from build123d import *

# Parameters (mm, degrees)
F1_DEPTH = 2.54
F2_R     = 1.651
F3_DEPTH = 25.4


with BuildPart() as f1:
    # F0 (on Front) → F1 (new body)
    with BuildSketch(Plane.XZ):
        with BuildLine():
            Line((-19.05, 0), (0, 0))
            Line((0, 0), (76.2, 0))
            ThreePointArc((76.2, 0), (100.04356, 25.4), (76.2, 50.8))
            Line((76.2, 50.8), (0, 50.8))
            Line((0, 50.8), (-19.05, 50.8))
            ThreePointArc((-19.05, 50.8), (-39.70724, 25.4), (-19.05, 0))
        make_face()
    extrude(amount=F1_DEPTH)

    # F2 (on face) → F3 (cut)
    with BuildSketch(Plane.XZ.offset(2.54)):
        with Locations((59.7933, 39.132159)):
            Circle(F2_R)
        with Locations((85.7267, 39.132159)):
            Circle(F2_R)
        with Locations((34.717675, 39.132159)):
            Circle(F2_R)
        with Locations((7.566978, 39.132159)):
            Circle(F2_R)
        with Locations((-13.534474, 39.132159)):
            Circle(F2_R)
    extrude(amount=-F3_DEPTH, mode=Mode.SUBTRACT)


solid = f1.part
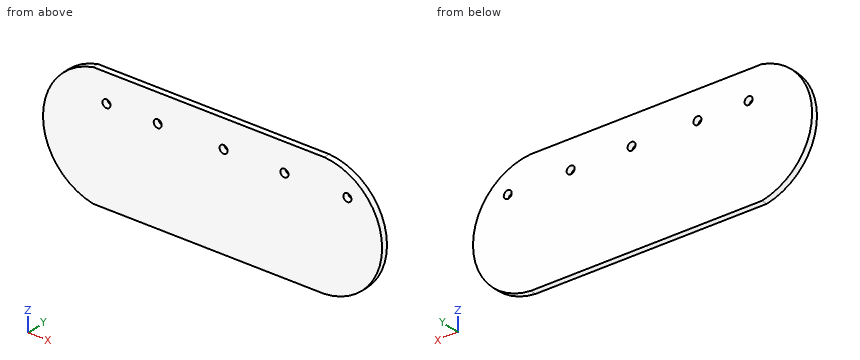
Geometry check sheet. Reference: the model listing, model coordinates, mm. Give positions to 0.01 mm unless a question says otherwise; leave off trailing zeros. Write each loop counter-clockwise with the first axis right and the second up, starting at its lowest first coordinate (ties: lowest second). Pieces come first, ordered by that corner, then holes. Notation, with made-up numbers: (10, 58) - (45, 58) arc R12 cw to (45, 78) - close; hole circle Ø9 at (49.5, -22). An arc over 180 degrees is marked (long way). Put each result on its own line as item: value.
1. Thickness scan on line 1 (X direction, y = -2.15, z = 40); line 2 (X direction, y = -1.3, z = 39); line 3 (Z direction, x = 86, y = -1.1). Record the ranges inside material, lowest first.
Ans:
line 1: x = -35.21 to -14.94, -12.13 to 6.16, 8.97 to 33.31, 36.12 to 58.39, 61.2 to 84.32, 87.13 to 95.44
line 2: x = -35.86 to -15.18, -11.89 to 5.92, 9.21 to 33.07, 36.36 to 58.15, 61.44 to 84.08, 87.37 to 96.11
line 3: z = 2.65 to 37.5, 40.76 to 48.15
2. Go/stop test with a flat-tipped pin: pin 1 (1.5 mm diameter, centred on y = -2, z = 42.5, fed in from +X). Record where the tip stops, or that it passes through.
Ans:
pin 1: stops at x = 94.1
3. Sectioned sample at A-A, the plane y = -1.95. Enter the section's corners in (x, z).
Ans:
outline: (-19.05, 0) - (76.2, 0) arc R25.45 ccw to (76.2, 50.8) - (-19.05, 50.8) arc R25.94 ccw to start; hole circle Ø3.3 at (-13.53, 39.13); hole circle Ø3.3 at (7.57, 39.13); hole circle Ø3.3 at (34.72, 39.13); hole circle Ø3.3 at (59.79, 39.13); hole circle Ø3.3 at (85.73, 39.13)
4. Sectioned sample at B-B, the plane z = 10. Enter the section's corners in (x, y), plus the area to 3 significant figures.
Ans:
outline: (-34.64, -2.54) - (94.86, -2.54) - (94.86, 0) - (-34.64, 0) - close
area: 329 mm²
5. Sectioned sample at C-C, the plane z = 44.5. Enter the section's corners in (x, y), plus the area to 3 significant figures.
Ans:
outline: (-31.32, -2.54) - (91.41, -2.54) - (91.41, 0) - (-31.32, 0) - close
area: 312 mm²
